from build123d import *

# Parameters (mm, degrees)
CYLINDER702_R               = 1.5
CYLINDER702_DEPTH           = 100
CYLINDER708_R               = 1.5
CYLINDER708_DEPTH           = 100
CYLINDER708_PLACEMENT_ANGLE = 145
CYLINDER699_R               = 1.5
CYLINDER699_DEPTH           = 100
CYLINDER707_R               = 1.5
CYLINDER707_DEPTH           = 100
CYLINDER707_PLACEMENT_ANGLE = 225
CYLINDER711_R               = 1.5
CYLINDER711_DEPTH           = 100
CYLINDER710_R               = 1.5
CYLINDER710_DEPTH           = 100
CYLINDER710_PLACEMENT_ANGLE = 45
CYLINDER701_R               = 1.5
CYLINDER701_DEPTH           = 100
CYLINDER701_PLACEMENT_ANGLE = 10
CYLINDER706_R               = 1.5
CYLINDER706_DEPTH           = 100
CYLINDER706_PLACEMENT_ANGLE = 45
CYLINDER713_R               = 8
CYLINDER713_DEPTH           = 18
CYLINDER704_R               = 8
CYLINDER704_DEPTH           = 18
CYLINDER704_PLACEMENT_ANGLE = 225
CYLINDER700_R               = 8
CYLINDER700_DEPTH           = 18
CYLINDER698_R               = 8
CYLINDER698_DEPTH           = 18
CYLINDER698_PLACEMENT_ANGLE = 145
CYLINDER712_R               = 8
CYLINDER712_DEPTH           = 18
CYLINDER709_R               = 8
CYLINDER709_DEPTH           = 18
CYLINDER709_PLACEMENT_ANGLE = 45
CYLINDER705_R               = 8
CYLINDER705_DEPTH           = 18
CYLINDER705_ROLL_ANGLE      = 0.146073
CYLINDER705_PITCH_ANGLE     = 1.079101
CYLINDER705_PLACEMENT_ANGLE = -9.939308
CYLINDER703_R               = 8
CYLINDER703_DEPTH           = 18
CYLINDER703_PLACEMENT_ANGLE = 45
TUBE076_R                   = 58
TUBE076_R_2                 = 30
TUBE076_DEPTH               = 8


with BuildPart() as obj1:
    # Cylinder702 → Cylinder702 (new body)
    with BuildSketch(Plane(origin=(38.80294, -16.072704, 0), x_dir=(0, 1, 0), z_dir=(0, 0, 1))):
        Circle(CYLINDER702_R)
    extrude(amount=CYLINDER702_DEPTH)


with BuildPart() as obj2:
    # Cylinder708 → Cylinder708 (new body)
    with BuildSketch(Plane.XY):
        Circle(CYLINDER708_R)
    extrude(amount=CYLINDER708_DEPTH)


with BuildPart() as obj2_1:
    # Cylinder708 placement: moved
    add(obj2.part.moved(Location((35.44, 22.53, 0.61))).rotate(Axis((35.44, 22.53, 0.61), (0, 0, 1)), CYLINDER708_PLACEMENT_ANGLE))


with BuildPart() as obj3:
    # Cylinder699 → Cylinder699 (new body)
    with BuildSketch(Plane(origin=(16.072704, 38.80294, 0), x_dir=(-1, 0, 0), z_dir=(0, 0, 1))):
        Circle(CYLINDER699_R)
    extrude(amount=CYLINDER699_DEPTH)


with BuildPart() as obj4:
    # Cylinder707 → Cylinder707 (new body)
    with BuildSketch(Plane.XY):
        Circle(CYLINDER707_R)
    extrude(amount=CYLINDER707_DEPTH)


with BuildPart() as obj4_1:
    # Cylinder707 placement: moved
    add(obj4.part.moved(Location((-16.072704, 38.80294, 0))).rotate(Axis((-16.072704, 38.80294, 0), (0, 0, 1)), CYLINDER707_PLACEMENT_ANGLE))


with BuildPart() as obj5:
    # Cylinder711 → Cylinder711 (new body)
    with BuildSketch(Plane(origin=(-38.80294, 16.072704, 0), x_dir=(0, -1, 0), z_dir=(0, 0, 1))):
        Circle(CYLINDER711_R)
    extrude(amount=CYLINDER711_DEPTH)


with BuildPart() as obj6:
    # Cylinder710 → Cylinder710 (new body)
    with BuildSketch(Plane.XY):
        Circle(CYLINDER710_R)
    extrude(amount=CYLINDER710_DEPTH)


with BuildPart() as obj6_1:
    # Cylinder710 placement: moved
    add(obj6.part.moved(Location((-38.80294, -16.072704, 0))).rotate(Axis((-38.80294, -16.072704, 0), (0, 0, -1)), CYLINDER710_PLACEMENT_ANGLE))


with BuildPart() as obj7:
    # Cylinder701 → Cylinder701 (new body)
    with BuildSketch(Plane.XY):
        Circle(CYLINDER701_R)
    extrude(amount=CYLINDER701_DEPTH)


with BuildPart() as obj7_1:
    # Cylinder701 placement: moved
    add(obj7.part.moved(Location((-22.53, -35.45, 0.2))).rotate(Axis((-22.53, -35.45, 0.2), (0, 0, 1)), CYLINDER701_PLACEMENT_ANGLE))


with BuildPart() as compound697:
    # Cylinder706 → Cylinder706 (new body)
    with BuildSketch(Plane.XY):
        Circle(CYLINDER706_R)
    extrude(amount=CYLINDER706_DEPTH)


with BuildPart() as compound697_1:
    # Cylinder706 placement: moved
    add(compound697.part.moved(Location((16.072704, -38.80294, 0))).rotate(Axis((16.072704, -38.80294, 0), (0, 0, 1)), CYLINDER706_PLACEMENT_ANGLE))

    # Compound697: union obj1, obj2, obj3, obj4, obj5, obj6, obj7
    add(obj1.part)
    add(obj2_1.part)
    add(obj3.part)
    add(obj4_1.part)
    add(obj5.part)
    add(obj6_1.part)
    add(obj7_1.part)


with BuildPart() as obj8:
    # Cylinder713 → Cylinder713 (new body)
    with BuildSketch(Plane(origin=(-38.798949, 16.072537, 43), x_dir=(0, -1, 0), z_dir=(0, 0, 1))):
        Circle(CYLINDER713_R)
    extrude(amount=CYLINDER713_DEPTH)


with BuildPart() as obj9:
    # Cylinder704 → Cylinder704 (new body)
    with BuildSketch(Plane.XY):
        Circle(CYLINDER704_R)
    extrude(amount=CYLINDER704_DEPTH)


with BuildPart() as obj9_1:
    # Cylinder704 placement: moved
    add(obj9.part.moved(Location((-16.07, 38.8, 43))).rotate(Axis((-16.07, 38.8, 43), (0, 0, 1)), CYLINDER704_PLACEMENT_ANGLE))


with BuildPart() as obj10:
    # Cylinder700 → Cylinder700 (new body)
    with BuildSketch(Plane(origin=(16.072537, 38.798949, 43), x_dir=(-1, 0, 0), z_dir=(0, 0, 1))):
        Circle(CYLINDER700_R)
    extrude(amount=CYLINDER700_DEPTH)


with BuildPart() as obj11:
    # Cylinder698 → Cylinder698 (new body)
    with BuildSketch(Plane.XY):
        Circle(CYLINDER698_R)
    extrude(amount=CYLINDER698_DEPTH)


with BuildPart() as obj11_1:
    # Cylinder698 placement: moved
    add(obj11.part.moved(Location((34.63, 22.64, 43.6))).rotate(Axis((34.63, 22.64, 43.6), (0, 0, 1)), CYLINDER698_PLACEMENT_ANGLE))


with BuildPart() as obj12:
    # Cylinder712 → Cylinder712 (new body)
    with BuildSketch(Plane(origin=(38.798949, -16.072537, 43), x_dir=(0, 1, 0), z_dir=(0, 0, 1))):
        Circle(CYLINDER712_R)
    extrude(amount=CYLINDER712_DEPTH)


with BuildPart() as obj13:
    # Cylinder709 → Cylinder709 (new body)
    with BuildSketch(Plane.XY):
        Circle(CYLINDER709_R)
    extrude(amount=CYLINDER709_DEPTH)


with BuildPart() as obj13_1:
    # Cylinder709 placement: moved
    add(obj13.part.moved(Location((16.07, -38.8, 43))).rotate(Axis((16.07, -38.8, 43), (0, 0, 1)), CYLINDER709_PLACEMENT_ANGLE))


with BuildPart() as obj14:
    # Cylinder705 → Cylinder705 (new body)
    with BuildSketch(Plane.XY):
        Circle(CYLINDER705_R)
    extrude(amount=CYLINDER705_DEPTH)


with BuildPart() as obj14_1:
    # Cylinder705 roll: moved
    add(obj14.part.rotate(Axis((0, 0, 0), (1, 0, 0)), CYLINDER705_ROLL_ANGLE))


with BuildPart() as obj14_2:
    # Cylinder705 pitch: moved
    add(obj14_1.part.rotate(Axis((0, 0, 0), (0, 1, 0)), CYLINDER705_PITCH_ANGLE))


with BuildPart() as obj14_3:
    # Cylinder705 placement: moved
    add(obj14_2.part.moved(Location((-21.748471, -35.690226, 43.196026))).rotate(Axis((-21.748471, -35.690226, 43.196026), (0, 0, 1)), CYLINDER705_PLACEMENT_ANGLE))


with BuildPart() as compound698:
    # Cylinder703 → Cylinder703 (new body)
    with BuildSketch(Plane.XY):
        Circle(CYLINDER703_R)
    extrude(amount=CYLINDER703_DEPTH)


with BuildPart() as compound698_1:
    # Cylinder703 placement: moved
    add(compound698.part.moved(Location((-38.8, -16.07, 43))).rotate(Axis((-38.8, -16.07, 43), (0, 0, -1)), CYLINDER703_PLACEMENT_ANGLE))

    # Compound698: union obj8, obj9, obj10, obj11, obj12, obj13, obj14
    add(obj8.part)
    add(obj9_1.part)
    add(obj10.part)
    add(obj11_1.part)
    add(obj12.part)
    add(obj13_1.part)
    add(obj14_3.part)


with BuildPart() as compound698_2:
    # Compound698 placement: moved
    add(compound698_1.part.moved(Location((0, 0, 12))))


with BuildPart() as obj15:
    # Tube076 → Tube076 (new body)
    with BuildSketch(Plane.XY.offset(52)):
        Circle(TUBE076_R)
        Circle(TUBE076_R_2, mode=Mode.SUBTRACT)
    extrude(amount=TUBE076_DEPTH)

    # Cut318: cut Compound698
    add(compound698_2.part, mode=Mode.SUBTRACT)

    # Cut319: cut Compound697
    add(compound697_1.part, mode=Mode.SUBTRACT)


solid = obj15.part
Geometry check sheet. Reference: the model listing, model coordinates, mm. A direction names the side the tool comes from. Round coordinates to 2 decimals unless told otherwise and drop trailing zeros. Order: outer loops, then holes, each group sorted by start corner. A loop starts at its lowest first (then second) coordinate and runs counter-clockwise, first axis right, second up. Notation, with made-up numbers: (-26.5, -28) -> (14.5, -28) arc R27 cw to (14.5, 8) -> close; hole circle Ø3 at (5, -30.75). An arc over 180 degrees is marked (long way). Use one line per item in the form item = value.
1. Scan lines: line 1 along X through (y, z) = (-15.5, 55.25); line 2 along X through (y, z) = (37.5, 58); line 3 along Y through (x, z) = (-16.07, 57.1). Record each from-to range of solid material in increasing order. Write a range as from..to.
Working result:
line_1 = -55.89..-46.78, -30.82..-25.69, 25.69..30.82, 46.78..55.89
line_2 = -44.25..-23.96, -8.18..8.18, 23.97..44.25
line_3 = -55.73..-41.37, -30.03..-25.33, 25.33..30.8, 46.8..55.73
2. Go/stop test with flat-tipped pins: pin 1 (5 mm diameter, centred on x = -38.5, y = -16, fed in from +Z); pin 2 (3 mm diameter, centred on y = 7, z = 58, fed in from +X); pin 3 (2.5 mm diameter, centred on x = -16.07, y = 38.8, fed in from -Z); pin 4 (1 mm diameter, centred on x = -24.5, z = 56, fed in from -Y). Record where each tip stops, or that it passes through.
Working result:
pin_1 = 55
pin_2 = 57.74
pin_3 = through
pin_4 = -52.8
3. Mould release check, pull along X, two halves, no side actions. Record for faces 3 (the face through (26.76, -51.46, 55.94)), 4 (the face through (25, -25, 52)), 5 (the face through (-21.36, -27.71, 57.68)), 6 (the face through (-29.97, 1.32, 55.94)): pulls with the +X half, pulls with the -X half, needs draft (parallel to the pull), parting line crosses it, or undercut.
Working result:
face_3 = parting line crosses it
face_4 = needs draft
face_5 = undercut
face_6 = undercut
4. Set-up check for faces 1 (the face through (-39.82, -14.97, 53.48)), 2 (the face through (-40.1, -17.2, 55)): record each of +Z, -Z, +X, -X, +Y, -Y from which the full face is reachable in a straight line by a thin tool's end or side.
Working result:
face_1 = +Z, -Z
face_2 = +Z
5. Cross-section at D-D, the plane y = 19. Enter the section's corners in (x, z).
Working result:
outline = (-54.8, 52) -> (-23.22, 52) -> (-23.22, 60) -> (-31.35, 60) -> (-31.35, 55) -> (-46.24, 55) -> (-46.24, 60) -> (-54.8, 60) -> close; (23.22, 52) -> (54.8, 52) -> (54.8, 60) -> (41.75, 60) -> (41.75, 55.6) -> (27.51, 55.6) -> (27.51, 60) -> (23.22, 60) -> close
6. Cross-section at C-C, the plane z = 53.75. Count the separate pieces of the cut face and the enclosed holes in it, plus the area to 3 significant figures.
Working result:
separate_pieces = 1
enclosed_holes = 9
area = 7,680 mm^2
7. Cross-section at A-A, the plane x = 0. Enter the section's corners in (y, z).
Working result:
outline = (-58, 52) -> (-30, 52) -> (-30, 60) -> (-58, 60) -> close; (30, 52) -> (58, 52) -> (58, 60) -> (30, 60) -> close
8. Cross-section at B-B, the plane y = 4. Enter the section's corners in (x, z).
Working result:
outline = (-57.86, 52) -> (-29.73, 52) -> (-29.73, 60) -> (-57.86, 60) -> close; (29.73, 52) -> (57.86, 52) -> (57.86, 60) -> (29.73, 60) -> close
